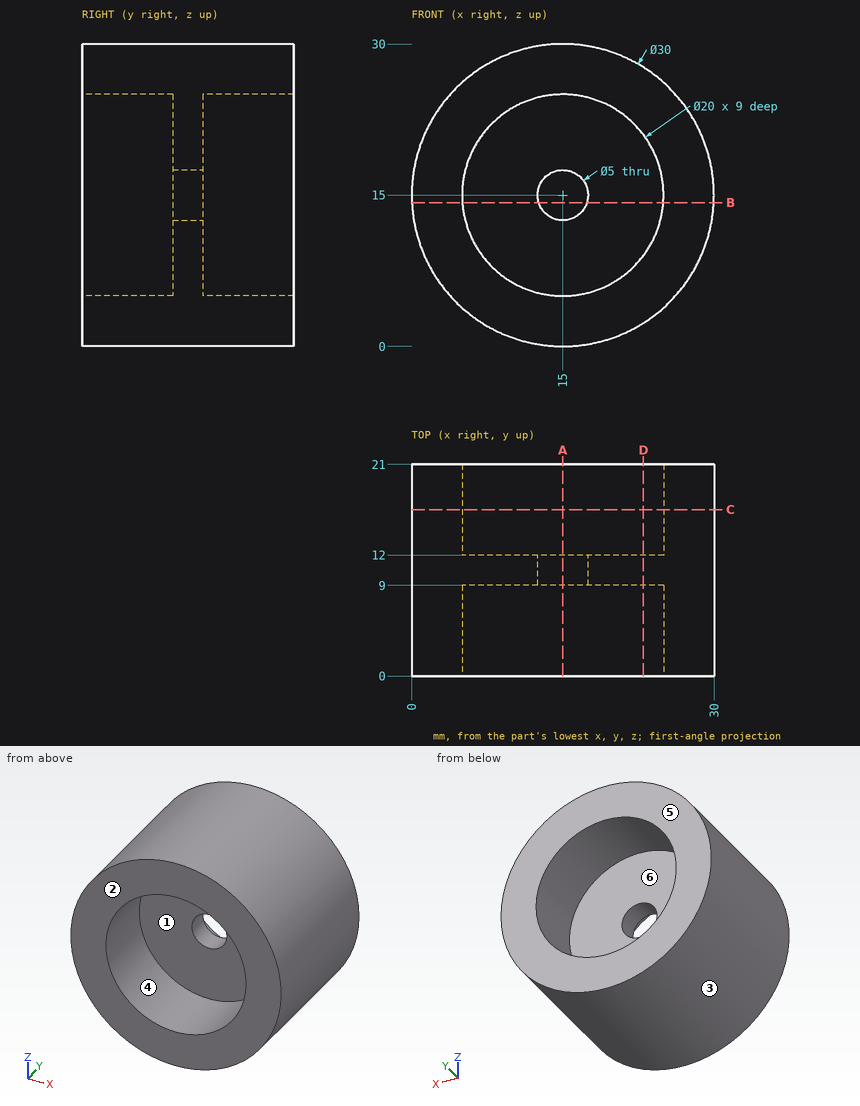
Drawing for the job (mm, zero at the part's lowest x, y, z). A direction names the side the tool comes from. Round coordinates to 2 decimals unless told otherwise and drop trailing zeros. Write each loop counter-clockwise with the first axis right and the second up, starting at its lowest first coordinate (ties: lowest second). Pieces come first, ordered by that corner, then holes. Notation, with made-up numbers: (11.25, -5) - (57.25, -5) arc R14 cw to (57.25, 9) - close; hole circle Ø3 at (16, 86). An arc over 180 degrees is marked (long way). Return JSON: item names as keys, results as strings. Group by question number.
Item 1: Band-saw the part on A-A on x = 15. List the corners of the cut face in (y, z).
Item 2: 3-axis set-ups, long thin cutter, end or side, ignore diameter. For the marked faces 4, 5 and 6: which of +Z, -Z, +X, -X, +Y, -Y reach the whole face in a straight line?
Item 3: Probe probe 1 along Z at (x, y) = (15, 17.75); probe 2 along Z at (x, y) = (15, 10.7); probe 3 along Y at (x, z) = (11.25, 13.25). List the from-to ranges inside material, lowest first.
Item 4: Band-saw the part on C-C on y = 16.5. List the corners of the cut face in (x, z).
Item 5: Band-saw the part on B-B on z = 14.25. List the corners of the cut face in (x, y), plus the area to 3 significant figures.
Item 6: Band-saw the part on D-D on x = 23. List the corners of the cut face in (y, z).
Item 7: Flat gauge pins, fed straight in: pin 1 Ø6.5 at (x, z) = (15, 15) entering from +Y; pin 2 Ø5 at (y, z) = (8.5, 5) entering from +X; pin 3 Ø8 at (x, y) = (7.5, 7) entering from -Z. Where does each tip first touch, or does it go through?
Item 8: Mould opens along X. For the marked faces 1, 2 and 3 say: +X half, -X half, draft (parallel to the pull), parting line (faces both ways), or undercut.
Resolved:
{
 "1": {"outline": "(0, 0) - (21, 0) - (21, 5) - (12, 5) - (12, 12.5) - (9, 12.5) - (9, 5) - (0, 5) - close; (0, 25) - (9, 25) - (9, 17.5) - (12, 17.5) - (12, 25) - (21, 25) - (21, 30) - (0, 30) - close"},
 "2": {"face 4": "-Y", "face 5": "+Z, -Z, +X, -X, +Y", "face 6": "+Y"},
 "3": {"probe 1": "z = 0 to 5, 25 to 30", "probe 2": "z = 0 to 12.5, 17.5 to 30", "probe 3": "y = 9 to 12"},
 "4": {"outline": "circle Ø30 at (15, 15); hole circle Ø20 at (15, 15)"},
 "5": {"outline": "(0.02, 0) - (5.03, 0) - (5.03, 9) - (12.62, 9) - (12.62, 12) - (5.03, 12) - (5.03, 21) - (0.02, 21) - close; (17.38, 9) - (24.97, 9) - (24.97, 0) - (29.98, 0) - (29.98, 21) - (24.97, 21) - (24.97, 12) - (17.38, 12) - close", "area": "256 mm²"},
 "6": {"outline": "(0, 2.31) - (21, 2.31) - (21, 9) - (12, 9) - (12, 21) - (21, 21) - (21, 27.69) - (0, 27.69) - (0, 21) - (9, 21) - (9, 9) - (0, 9) - close"},
 "7": {"pin 1": "stops at y = 12", "pin 2": "stops at x = 27.99", "pin 3": "stops at z = 0.41"},
 "8": {"face 1": "undercut", "face 2": "draft", "face 3": "parting line"}
}
